```python
from build123d import *

# Parameters (mm, degrees)
F0_R     = 10.16
F0_R_2   = 5.08
F1_DEPTH = 6.35
F0_R_3   = 2.54
F2_DEPTH = 5.08


with BuildPart() as f1:
    # F0 (on Top) → F1 (new body)
    with BuildSketch(Plane.XY):
        Circle(F0_R)
        Circle(F0_R_2, mode=Mode.SUBTRACT)
    extrude(amount=F1_DEPTH)



with BuildPart() as f1b:
    # F0 (on Top) → F1, piece 2 (new body)
    with BuildSketch(Plane.XY):
        Circle(F0_R_3)
    extrude(amount=F1_DEPTH)


with BuildPart() as f1_1:
    add(f1.part)

    add(f1b.part)  # F2 merges F1b
    # F0 (on Top) → F2 (join)
    with BuildSketch(Plane.XY):
        Circle(F0_R)
        Circle(F0_R_2, mode=Mode.SUBTRACT)
        Circle(F0_R_2)
        Circle(F0_R_3, mode=Mode.SUBTRACT)
    extrude(amount=F2_DEPTH)


solid = f1_1.part
```
Work out the finished part from the listing and answer in its coordinate system (mm). A direction names the side the tool comes from. Coordinates: 2 decimals unless noted, no trailing zeros. Write each loop counter-clockwise with the first axis right and the second up, starting at its lowest first coordinate (ties: lowest second). Pieces come first, ordered by that corner, then holes. Notation, with made-up numbers: (-25.75, -7.5) - (28.25, -7.5) arc R28 ccw to (28.25, 23.5) - close; hole circle Ø7 at (16, 16). An arc over 180 degrees is marked (long way). Answer as a JSON object with one key per item and string values.
Q1. Find section D-D (y = -3.25). Write down the section's boundary in (x, z), plus the area to 3 significant figures.
Results list:
{"outline": "(-9.63, 0) - (9.63, 0) - (9.63, 6.35) - (3.9, 6.35) - (3.9, 5.08) - (-3.9, 5.08) - (-3.9, 6.35) - (-9.63, 6.35) - close", "area": "112 mm^2"}
Q2. Given pin 1 Ø1 at (x, z) = (-8, 4.5) entering from +Y; pin 2 Ø1.5 at (y, z) = (-2.5, 3.5) entering from -X; pin 3 Ø1.5 at (x, z) = (-8, 1.5) entering from -Y, each flat-ended and moving along its own axis, determine where each tip first touches the part or whether it passes through.
Results list:
{"pin 1": "stops at y = 6.85", "pin 2": "stops at x = -10.01", "pin 3": "stops at y = -7.12"}
Q3. Consider L1, parallel to Y at x = 0, z = 6.05; L2, parallel to X at y = 1.5, z = 6.25; L3, parallel to Z at x = 3.5, y = 3.25. Determine where each line is inside the solid, lowest interval first. Write a range as from..to.
Results list:
{"L1": "y = -10.16..-5.08, -2.54..2.54, 5.08..10.16", "L2": "x = -10.05..-4.85, -2.05..2.05, 4.85..10.05", "L3": "z = 0..5.08"}
Q4. Which of the six approach directions +Z, -Z, +X, -X, +Y, -Y give full straight-line access (tool end or side, diameter ignored) to faces 4 (the flat face through (2, -2, 5.08)), 5 (the flat face through (0, 0, 0))?
Results list:
{"face 4": "+Z", "face 5": "-Z, +X, -X, +Y, -Y"}
Q5. For a pull along X with two mould halves and no side action, classify faces 1 (the flat face through (-5, -2, 6.35)), 2 (the cylindrical face through (-0.661, 5.037, 5.706)), 3 (the cylindrical face through (-1.323, 10.074, 3.131)) as pulls with the +X half, pulls with the -X half, needs draft (parallel to the pull), parting line crosses it, or undercut.
Results list:
{"face 1": "needs draft", "face 2": "undercut", "face 3": "parting line crosses it"}
Q6. Find section C-C (z = 4.75). Write down the section's boundary in (x, y), plus the area to 3 significant figures.
Results list:
{"outline": "circle Ø20.32 at (0, 0)", "area": "324 mm^2"}
Q7. Find section A-A (y = 0). Write down the section's boundary in (x, z).
Results list:
{"outline": "(-10.16, 0) - (10.16, 0) - (10.16, 6.35) - (5.08, 6.35) - (5.08, 5.08) - (2.54, 5.08) - (2.54, 6.35) - (-2.54, 6.35) - (-2.54, 5.08) - (-5.08, 5.08) - (-5.08, 6.35) - (-10.16, 6.35) - close"}
